Check sheet for the drawn part. Datum: minimum x, y, z corner. Units: mm. Give positions to 0.01 mm unless a question says otherwise; leave off trailing zeros. Order: outer loops, then holes, each group sorted by start corner. A loop starts at its lowest first (then second) coordinate and runs counter-clockwise, first axis right, second up. Notation, with made-up numbers: (58.25, 21.5) -> (71.25, 21.5) arc R30 ccw to (71.25, 52.5) -> close; hole circle Ø9 at (14.5, 45). An arc over 180 degrees is marked (long way). Return JSON: item names as keys, results as strings. Group by question number.
(1) Release check for a two-part mould opening along Y. For the marked faces 1 and 2 record: pulls with the +Y half, pulls with the -Y half, needs draft (parallel to the pull), parting line crosses it, or undercut.
(2) Depth check by flat-ended pin: pin 1 Ø3 at (x, z) = (8.5, 16.5) entering from -Y; pin 2 Ø4 at (y, z) = (3, 22.5) entering from +X; pin 3 Ø1.5 at (x, z) = (4.5, 25) entering from +Y. Enter the tip coordinate at first touch or a pass-through.
(3) Cross-section at A-A on z = 4. Enter the section's corners in (x, y).
(4) Cross-section at C-C on x = 11.25. Enter the section's corners in (y, z).
(5) Cross-section at B-B on y = 1.25. Enter the section's corners in (x, z), then the cut area to 3 significant figures.
(6) Thickness scan on line 1 along X through (y, z) = (5.75, 28); line 2 along Y through (x, z) = (2.5, 16). Record the ranges inside material, lowest first.
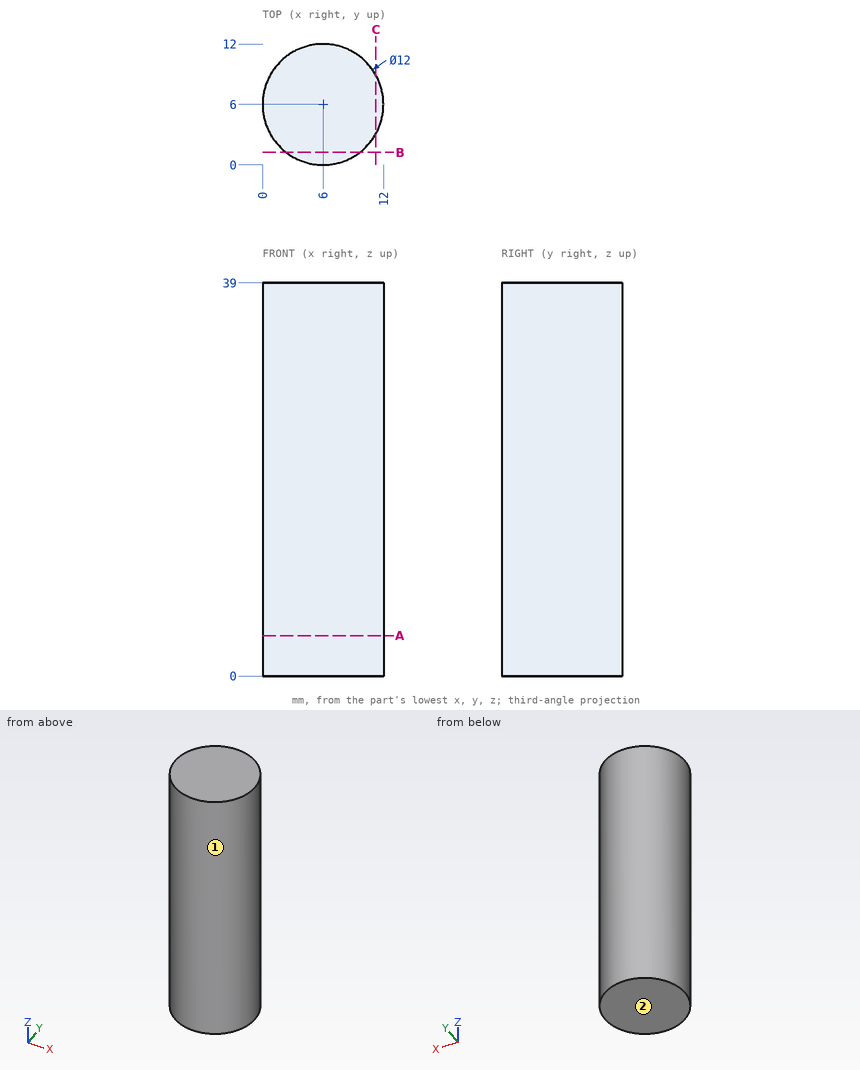
Verdict:
{
 "1": {"face 1": "parting line crosses it", "face 2": "needs draft"},
 "2": {"pin 1": "y = 0.08", "pin 2": "x = 11.92", "pin 3": "y = 11.95"},
 "3": {"outline": "circle Ø12 at (6, 6)"},
 "4": {"outline": "(3.1, 0) -> (8.9, 0) -> (8.9, 39) -> (3.1, 39) -> close"},
 "5": {"outline": "(2.33, 0) -> (9.67, 0) -> (9.67, 39) -> (2.33, 39) -> close", "area": "286 mm²"},
 "6": {"line 1": "0.01 to 11.99", "line 2": "1.13 to 10.87"}
}
